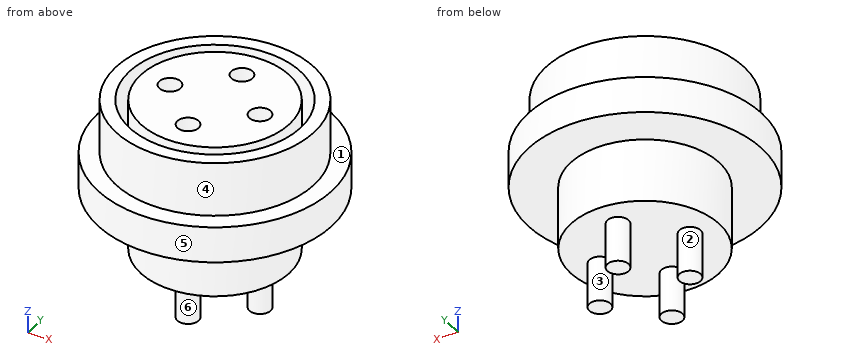
Autodesk Inventor part; units mm, degrees
ref_plane "YZ Plane" through (0, 0, 0) normal (1, 0, 0) x (0, 1, 0)
ref_plane "XZ Plane" through (0, 0, 0) normal (0, 1, 0) x (-1, 0, 0)
ref_plane "XY Plane" through (0, 0, 0) normal (0, 0, 1) x (1, 0, 0)
sketch "Sketch1" plane through (0, 0, 0) normal (0, 0, 1) x (1, 0, 0)
  circle A0 centre (0, 0) radius 10.5
  dimension "d0" = 21
extrude "Extrusion1" add sketch "Sketch1" along normal blind 8.89
sketch "Sketch2" plane through (0, 0, 8.89) normal (0, 0, 1) x (1, 0, 0)
  circle A0 centre (0, 0) radius 16.51
  dimension "d3" = 33.02
extrude "Extrusion2" add sketch "Sketch2" along normal blind 5.08
sketch "Sketch3" plane through (0, 0, 13.97) normal (0, 0, 1) x (1, 0, 0)
  circle A0 centre (0, 0) radius 13.97
  dimension "d6" = 27.94
extrude "Extrusion3" add sketch "Sketch3" along normal blind 7.62
sketch "Sketch4" plane through (0, 0, 21.59) normal (0, 0, 1) x (1, 0, 0)
  circle A0 centre (0, 0) radius 6.35 construction
  circle A1 centre (0, 6.35) radius 1.5
  circle A2 centre (-6.35, 0) radius 1.5
  circle A3 centre (0, -6.35) radius 1.5
  circle A4 centre (6.35, 0) radius 1.5
  dimension "d9" = 12.7
  dimension "d10" = 3
  dimension "d13" = 360
extrude "Extrusion4" cut sketch "Sketch4" against normal blind 11.43
sketch "Sketch5" plane through (0, 0, 21.59) normal (0, 0, 1) x (1, 0, 0)
  circle A0 centre (0, 0) radius 10.5
  circle A1 centre (0, 0) radius 10.5
  circle A2 centre (0, 0) radius 12.065
  dimension "d17" = 24.13
extrude "Extrusion5" cut sketch "Sketch5" against normal blind 11.43
sketch "Sketch6" plane through (0, 0, 0) normal (0, 0, -1) x (-1, 0, 0)
  circle A0 centre (0, 6.35) radius 1.5
  circle A1 centre (0, 0) radius 6.35 construction
  circle A2 centre (0, 6.35) radius 1.5
  circle A3 centre (0, 0) radius 6.35 construction
  circle A4 centre (-6.35, 0) radius 1.5
  circle A5 centre (0, 0) radius 6.35 construction
  circle A6 centre (0, -6.35) radius 1.5
  circle A7 centre (0, 0) radius 6.35 construction
  circle A8 centre (6.35, 0) radius 1.5
  dimension "d22" = 360
extrude "Extrusion6" add sketch "Sketch6" along normal blind 6.35
properties part number "connector" material "Rubber"
Could you check a few things on this model? Use its own coordinates, in mm. Face numbers are marked on the shaded views. A direction names the side the tool comes from. Round coordinates to 2 decimals unless told otherwise and drop trailing zeros. Write each loop counter-clockwise with the first axis right and the second up, starting at its lowest first coordinate (ties: lowest second). Pieces come first, ordered by that corner, then holes. Notation, with made-up numbers: M 12.25,83 L 57.25,83 A20 cw 57.25,112 Z; hole C 83,-3.5 d2. An arc over 180 degrees is marked long. Write each question's results on one line, items separated by ' | '. Start each with the question number.
1. I need wall thicknesses on L1, parallel to Y at x = 0, z = 19.25 (3 decimals); L2, parallel to Y at x = -6, z = 18.75; L3, parallel to Y at x = 6.35, z = 13.25. Which ranges of each line are inside material? Lowest first, please. Write a range as from..to.
2. On a 3-axis mill with a long thin cutter (end or side, diameter ignored), from which of +Z, -Z, +X, -X, +Y, -Y can I reach the whole of each face in a straight line? I mean the marked faces 5 and 6. Say none if no direction works.
3. I'm going to push flat-ended pins straight in: pin 1 Ø5 at (x, z) = (1, 16.5) entering from +Y; pin 2 Ø5 at (x, z) = (-7, 3.5) entering from +Y; pin 3 Ø0.9 at (x, y) = (0, -6.5) entering from +Z. Where does each tip first touch, or does it pass through?
4. Imagine slicing it at B-B on z = 17.5. List the corners of the cut face in (x, y) for me (3 decimals).
5. Imagine slicing it at A-A on z = 12.5. List the corners of the cut face in (x, y) for me (3 decimals).
6. Imagine slicing it at D-D on z = -2. List the corners of the cut face in (x, y) for me.
7. Thinking about a two-plate mould opening in X: for the marked faces 1, 2, 3 and 4, which applies, +X half, -X half, draft (parallel to the pull), parting line (faces both ways), or undercut?
8. Imagine slicing it at C-C on x = -4. List the corners of the cut face in (y, z) for me.
Result sheet:
1) L1: y = -13.97..-12.065, -10.5..-7.85, -4.85..4.85, 7.85..10.5, 12.065..13.97 | L2: y = -12.62..-10.47, -8.62..-1.46, 1.46..8.62, 10.47..12.62 | L3: y = -15.24..-10.26, -8.36..-1.5, 1.5..8.36, 10.26..15.24
2) face 5: +Z, -Z | face 6: -Z
3) pin 1: stops at y = 13.97 | pin 2: stops at y = 9.49 | pin 3: stops at z = 10.16
4) outline: C 0,0 d27.94; C 0,0 d21; hole C 0,0 d24.13; hole C -6.35,0 d3; hole C 0,-6.35 d3; hole C 0,6.35 d3; hole C 6.35,0 d3
5) outline: C 0,0 d33.02; C 0,0 d21; hole C 0,0 d24.13; hole C -6.35,0 d3; hole C 0,-6.35 d3; hole C 0,6.35 d3; hole C 6.35,0 d3
6) outline: C -6.35,0 d3; C 0,-6.35 d3; C 0,6.35 d3; C 6.35,0 d3
7) face 1: draft | face 2: undercut | face 3: undercut | face 4: parting line
8) outline: M -16.02,8.89 L -9.71,8.89 L -9.71,0 L 9.71,0 L 9.71,8.89 L 16.02,8.89 L 16.02,13.97 L 13.39,13.97 L 13.39,21.59 L 11.38,21.59 L 11.38,10.16 L 9.71,10.16 L 9.71,21.59 L -9.71,21.59 L -9.71,10.16 L -11.38,10.16 L -11.38,21.59 L -13.39,21.59 L -13.39,13.97 L -16.02,13.97 Z
